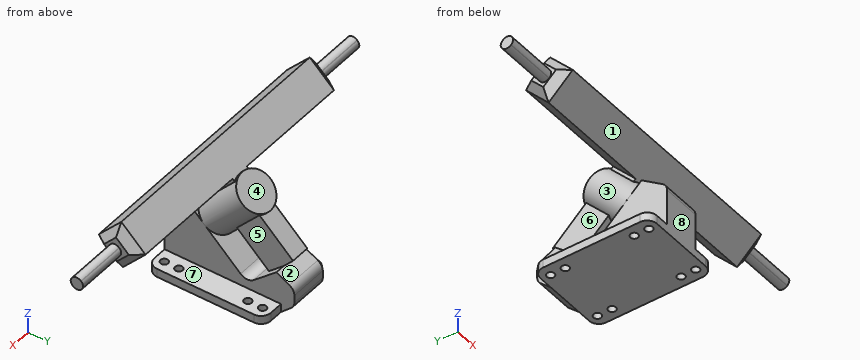
from build123d import *

# Parameters (mm, degrees)
F0_R      = 2.49555
F1_DEPTH  = 5.4991
F3_DEPTH  = 12.6365
F4_R      = 12.7
F5_DEPTH  = 36.195
F8_DEPTH  = 21.59
F7_W      = 33.9344
F7_H      = 7.9375
F9_DEPTH  = 13.4493
F10_DEPTH = 5.5118
F11_SIZE  = 5.08
F12_R     = 3.81


with BuildPart() as f1:
    # F0 (on Top) → F1 (new body)
    with BuildSketch(Plane.XY):
        with BuildLine():
            Line((21.6535, 38.00475), (-21.6535, 38.00475))
            ThreePointArc((-21.6535, 38.00475), (-26.1436280605, 36.1448780605), (-28.0035, 31.65475))
            Line((-28.0035, 31.65475), (-28.0035, -31.65475))
            ThreePointArc((-28.0035, -31.65475), (-26.1436280605, -36.1448780605), (-21.6535, -38.00475))
            Line((-21.6535, -38.00475), (21.6535, -38.00475))
            ThreePointArc((21.6535, -38.00475), (26.1436280605, -36.1448780605), (28.0035, -31.65475))
            Line((28.0035, -31.65475), (28.0035, 31.65475))
            ThreePointArc((28.0035, 31.65475), (26.1436280605, 36.1448780605), (21.6535, 38.00475))
        make_face()
        with Locations((-20.68195, -32.0802)):
            Circle(F0_R, mode=Mode.SUBTRACT)
        with Locations((-20.68195, -22.5171)):
            Circle(F0_R, mode=Mode.SUBTRACT)
        with Locations((20.94865, -32.0802)):
            Circle(F0_R, mode=Mode.SUBTRACT)
        with Locations((20.94865, -22.5171)):
            Circle(F0_R, mode=Mode.SUBTRACT)
        with Locations((-20.68195, 22.5171)):
            Circle(F0_R, mode=Mode.SUBTRACT)
        with Locations((-20.68195, 32.0802)):
            Circle(F0_R, mode=Mode.SUBTRACT)
        with Locations((20.94865, 22.5171)):
            Circle(F0_R, mode=Mode.SUBTRACT)
        with Locations((20.94865, 32.0802)):
            Circle(F0_R, mode=Mode.SUBTRACT)
    extrude(amount=F1_DEPTH)

    # F2 (on Right) → F3 (join, symmetric)
    with BuildSketch(Plane.YZ):
        with BuildLine():
            Line((-38.00475, 0), (38.00475, 0))
            Line((38.00475, 0), (44.6684117025, 6.0475273605))
            ThreePointArc((44.6684117025, 6.0475273605), (46.2070110218, 8.1783938925), (46.7509385842, 10.7497792875))
            Line((46.7509385842, 10.7497792875), (46.7509385842, 15.6225843746))
            ThreePointArc((46.7509385842, 15.6225843746), (45.8705955509, 18.8483172628), (43.4736621539, 21.1796402376))
            Line((43.4736621539, 21.1796402376), (35.0811212719, 25.8202194964))
            Line((35.0811212719, 25.8202194964), (20.0922738228, 12.9981952029))
            ThreePointArc((20.0922738228, 12.9981952029), (15.826745806, 11.4750322558), (11.6312994892, 13.1817791111))
            Line((11.6312994892, 13.1817791111), (-21.3543212783, 43.9746556756))
            Line((-21.3543212783, 43.9746556756), (-35.2473775709, 34.4420485715))
            ThreePointArc((-35.2473775709, 34.4420485715), (-37.2732767231, 32.1648917383), (-38.00475, 29.2060646967))
            Line((-38.00475, 29.2060646967), (-38.00475, 0))
        make_face()
    extrude(amount=F3_DEPTH, both=True)

    # F4 (on face) → F5 (join)
    with BuildSketch(Plane(origin=(0, 11.9915573283, 12.8454696856), x_dir=(1, 0, 0), z_dir=(0, 0.6823928283, 0.7309856551))):
        with Locations((0, -32.9176921867)):
            Circle(F4_R)
    extrude(amount=F5_DEPTH)

    # F7 (on offset) → F8 (join)
    with BuildSketch(Plane(origin=(0, 20.6579462472, 22.1289875052), x_dir=(1, 0, 0), z_dir=(0, 0.6823928283, 0.7309856551))):
        Polygon((6.35, 5.7192138057), (6.35, 8.0242638057), (-6.35, 8.0242638057), (-6.35, 5.7192138057), (-6.35, -45.9507361943), (-57.15, -45.9507361943), (-88.9, -45.9507361943), (-88.9, -52.7769861943), (-88.9, -60.7144861943), (-88.9, -67.5407361943), (0, -67.5407361943), (88.9, -67.5407361943), (88.9, -60.7144861943), (88.9, -52.7769861943), (88.9, -45.9507361943), (57.15, -45.9507361943), (6.35, -45.9507361943), align=None)
    extrude(amount=F8_DEPTH)

    # F7 (on offset) → F9 (join)
    with BuildSketch(Plane(origin=(0, 20.6579462472, 22.1289875052), x_dir=(1, 0, 0), z_dir=(0, 0.6823928283, 0.7309856551))):
        with Locations((105.8672, -56.7457361943)):
            Rectangle(F7_W, F7_H)
        with Locations((-105.8672, -56.7457361943)):
            Rectangle(F7_W, F7_H)
    extrude(amount=F9_DEPTH)

    # F7 (on offset) → F10 (cut)
    with BuildSketch(Plane(origin=(0, 20.6579462472, 22.1289875052), x_dir=(1, 0, 0), z_dir=(0, 0.6823928283, 0.7309856551))):
        with Locations((105.8672, -56.7457361943)):
            Rectangle(F7_W, F7_H)
        with Locations((-105.8672, -56.7457361943)):
            Rectangle(F7_W, F7_H)
    extrude(amount=F10_DEPTH, mode=Mode.SUBTRACT)

    # F11
    f11_edges = [f1.edges().sort_by_distance(p)[0] for p in [
        (88.9, -21.346932, 76.109292),
        (88.9, -6.089512, 76.633851),
        (88.9, -5.564952, 61.37643),
        (88.9, -20.822373, 60.851871),
        (-88.9, -6.089512, 76.633851),
        (-88.9, -21.346932, 76.109292),
        (-88.9, -5.564952, 61.37643),
        (-88.9, -20.822373, 60.851871),
    ]]
    chamfer(f11_edges, length=F11_SIZE)

    # F12
    f12_edges = [f1.edges().sort_by_distance(p)[0] for p in [
        (105.8672, -14.545766, 73.391363),
        (105.8672, -19.962259, 67.589164),
        (105.8672, -14.160061, 62.172671),
        (105.8672, -8.743568, 67.97487),
        (-105.8672, -19.962259, 67.589164),
        (-105.8672, -14.545766, 73.391363),
        (-105.8672, -8.743568, 67.97487),
        (-105.8672, -14.160061, 62.172671),
    ]]
    fillet(f12_edges, radius=F12_R)


solid = f1.part
Geometry: final body of the model. Coordinates: model frame, mm. Face numbers are marked on the shaded views. A direction names the side the tool comes from. Give positions to 0.01 mm unless a question says otherwise; leave off trailing zeros. Loops run counter-clockwise (first coordinate to the right, second up) from the corner with the lowest first, then second, coordinate; pieces in that order, holes last. Notation, with made-up numbers: (-15, 40.25) - (1, 40.25) arc R17 ccw to (1, 46.25) - close; hole circle Ø7 at (87.5, -20). An arc over 180 degrees is marked (long way). Answer as CSV lines item,"result". Start each with the question number.
1. Ray query, L1, parallel to Z at x = -23.5, y = 24; L2, parallel to X at y = -18.5, z = 34; L3, parallel to X at y = -4, z = 4. Return the intervals inside material, ascending.
2. Draft query along Y for the marked faces 1, 2 and 3. Return one class per face: released by +Y, released by -Y, zero draft, split by the parting line, or undercut.
3. Section A-A, the plane x = 15.5. Return loops of the section in (y, z), plus the area to 3 significant figures.
4. Section B-B, the plane z = 79.5. Return loops of the section in (x, y).
5. Section C-C, the plane x = 53.5. Return loops of the section in (y, z), plus the area to 3 significant figures.
6. Pin query (flat end, axial travel): P1, Ø17, axis at x = 17.5, y = -4, coming from the +Z side; P2, Ø4.5, axis at x = -20.68, y = 22.52, coming from the -Z side; P3, Ø22, axis at y = 23.5, z = 29.5, coming from the +X side; P4, Ø8, axis at x = 40, z = 60, coming from the +Y side. Return the tip coordinate at first contact, or that it passes through.
7. Reachability of the marked faces 4, 5, 6, 7 and 8 from +Z, -Z, +X, -X, +Y, -Y: full face, straight path, thin tool, end or side. Return the list, or none.
Answers:
1,L1,"z = 0 to 5.5"
1,L2,"x = -12.64 to 12.64"
1,L3,"x = -28 to 28"
2,face 1,"released by -Y"
2,face 2,"released by +Y"
2,face 3,"undercut"
3,outline,"(-38, 0) - (38, 0) - (38, 5.5) - (-38, 5.5) - close; (-28.71, 68.22) - (-12.93, 53.49) - (1.8, 69.27) - (-13.98, 84) - close"
3,area,"884 mm2"
4,outline,"(-87, -13.83) - (-83.82, -18.18) - (83.82, -18.18) - (87, -13.83) - (83.82, -9.16) - (-83.82, -9.16) - close"
5,outline,"(-28.71, 68.22) - (-12.93, 53.49) - (1.8, 69.27) - (-13.98, 84) - close"
5,area,"466 mm2"
6,P1,"stops at z = 82.62"
6,P2,"passes through"
6,P3,"stops at x = 12.64"
6,P4,"stops at y = -3.12"
7,face 4,"+Z, +X, -X, +Y"
7,face 5,"+X"
7,face 6,"-X"
7,face 7,"+X, +Y, -Y"
7,face 8,"+Z, -Z, +X, -X, -Y"
